Read the model definition and answer for the solid it produces. Units are mm, in the model's axes. Face numbers are marked on the shaded views. Round coordinates to 2 decimals unless told otherwise and drop trailing zeros. Order: outer loops, then holes, each group sorted by start corner. A loop starts at its lowest first (then second) coordinate and runs counter-clockwise, first axis right, second up. Notation, with made-up numbers: (52.25, 39) -> (107.25, 39) arc R23 cw to (107.25, 64) -> close; hole circle Ø7 at (46.25, -37). An arc over 180 degrees is marked (long way). One line per item, written item: value. Start each with the question number.
1. Consider line 1 (Y direction, x = 0, z = 2.2) (3 decimals); line 2 (Y direction, x = 0, z = 5.25) (1 decimal); line 3 (X direction, y = 32.5, z = 8.75). Determine where each line is inside the solid, lowest interval first.
2. Section D-D (y = 23) is taken. Give the vertices of the cut face in (x, z) (3 decimals).
3. Section B-B (x = 0) is taken. Give the vertices of the cut face in (y, z) (1 decimal), then the cut area to 3 significant figures.
4. Section C-C (z = 8) is taken. Give the vertices of the cut face in (x, y) (1 decimal).
5. The mould has two halves that part along Y. Classify the marked faces 1 and 2: released by +Y, released by -Y, zero draft, split by the parting line, or undercut.
6. Section A-A (y = 0) is taken. Give the vertices of the cut face in (x, z) (1 decimal), then the cut area to 3 significant figures.
7. Flat-ended cylindrical pins translate along their axes: pin 1 Ø5 at (y, z) = (43.5, 3.5) entering from -X; pin 2 Ø5 at (x, z) = (-54, 5.5) entering from +Y; pin 3 Ø1 at (y, z) = (-36.5, 5.5) entering from -X; pin 4 Ø11.5 at (x, y) = (98.425, 0) entering from +Z (3 decimals). Find the tip coordinate at first contact, or state that the pin passes through.
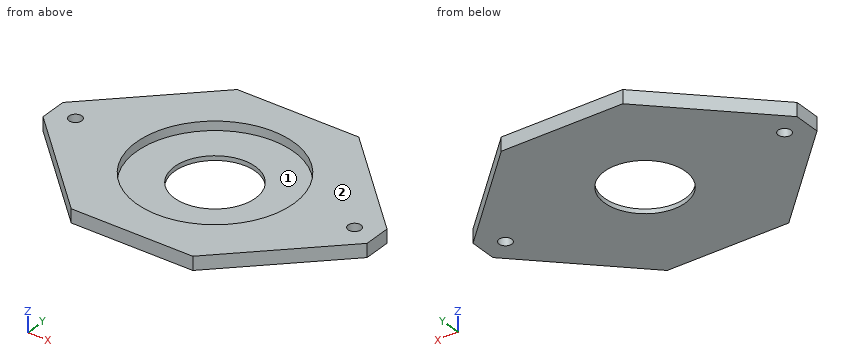
from build123d import *

# Parameters (mm, degrees)
F1_DEPTH = 9.525
F2_R     = 55.5625
F3_DEPTH = 6.35
F5_D     = 9
F6_R     = 28.575
F7_DEPTH = 3.176


with BuildPart() as f1:
    # F0 (on Top) → F1 (new body)
    with BuildSketch(Plane.XY):
        Polygon((-42.8625, 79.375), (-114.3, 9.525), (-114.3, -9.525), (-42.8625, -79.375), (42.8625, -79.375), (114.3, -9.525), (114.3, 9.525), (42.8625, 79.375), align=None)
    extrude(amount=F1_DEPTH)

    # F2 (on face) → F3 (cut)
    with BuildSketch(Plane.XY.offset(9.525)):
        Circle(F2_R)
    extrude(amount=-F3_DEPTH, mode=Mode.SUBTRACT)

    # F5 (through all)
    with Locations(Plane.XY.offset(9.525)):
        with Locations((-98.425, 0), (98.425, 0)):
            Hole(F5_D / 2)

    # F6 (on face) → F7 (cut, through all)
    with BuildSketch(Plane.XY.offset(3.175)):
        Circle(F6_R)
    extrude(amount=-F7_DEPTH, mode=Mode.SUBTRACT)


solid = f1.part
Answer:
1. line 1: -79.375 to -28.575, 28.575 to 79.375
1. line 2: -79.4 to -55.6, 55.6 to 79.4
1. line 3: -90.8 to -45.07, 45.07 to 90.8
2. outline: (-100.519, 0) -> (-16.957, 0) -> (-16.957, 3.175) -> (-50.579, 3.175) -> (-50.579, 9.525) -> (-100.519, 9.525) -> close; (16.957, 0) -> (100.519, 0) -> (100.519, 9.525) -> (50.579, 9.525) -> (50.579, 3.175) -> (16.957, 3.175) -> close
3. outline: (-79.4, 0) -> (-28.6, 0) -> (-28.6, 3.2) -> (-55.6, 3.2) -> (-55.6, 9.5) -> (-79.4, 9.5) -> close; (28.6, 0) -> (79.4, 0) -> (79.4, 9.5) -> (55.6, 9.5) -> (55.6, 3.2) -> (28.6, 3.2) -> close
3. area: 625 mm^2
4. outline: (-114.3, -9.5) -> (-42.9, -79.4) -> (42.9, -79.4) -> (114.3, -9.5) -> (114.3, 9.5) -> (42.9, 79.4) -> (-42.9, 79.4) -> (-114.3, 9.5) -> close; hole circle Ø9 at (-98.4, 0); hole circle Ø111.1 at (0, 0); hole circle Ø9 at (98.4, 0)
5. face 1: undercut
5. face 2: zero draft
6. outline: (-114.3, 0) -> (-102.9, 0) -> (-102.9, 9.5) -> (-114.3, 9.5) -> close; (-93.9, 0) -> (-28.6, 0) -> (-28.6, 3.2) -> (-55.6, 3.2) -> (-55.6, 9.5) -> (-93.9, 9.5) -> close; (28.6, 0) -> (93.9, 0) -> (93.9, 9.5) -> (55.6, 9.5) -> (55.6, 3.2) -> (28.6, 3.2) -> close; (102.9, 0) -> (114.3, 0) -> (114.3, 9.5) -> (102.9, 9.5) -> close
6. area: 1,120 mm^2
7. pin 1: x = -82.11
7. pin 2: y = 70.93
7. pin 3: x = -87.22
7. pin 4: z = 9.525
